Source: three-view drawing plus pictorial views. Frame: mm from the lowest corner of the part. A direction names the side the tool comes from. Give positions to 0.01 mm unless a question says otherwise; leave off trailing zeros. Loops run counter-clockwise (first coordinate to the right, second up) from the corner with the lowest first, then second, coordinate; pieces in that order, holes last. Notation, with made-up numbers: M -18,24 L -14,24 A32 ccw -14,58 Z; hole C 62,65 d8. An arc over 180 degrees is marked long. One line per item, written item: value. Start each with the question number.
(1) Section C-C on z = 16.5. Output: boundary loops of the cut face in (x, y), plus the area to 3 significant figures.
(2) Pin query (flat end, axial travel): P1, Ø4, axis at x = 6, y = 3, coming from the +Z side; P2, Ø2.5, axis at x = 5.5, y = 7, coming from the +Z side; P3, Ø2.5, axis at y = 1.5, z = 13, coming from the -X side; P4, Ø6, axis at x = 6.5, z = 11.5, coming from the -Y side. Return the tip coordinate at first contact, or that it passes through.
(3) Pull-direction query (Z, two-part tool) for the marked faces 1, 2, 3 and 4; classes: released by +Z, released by -Z, zero draft, split by the parting line, or undercut.
(4) Access query for the marked faces 5, 6, 7, 8 and 9. Directions: +Z, -Z, +X, -X, +Y, -Y. A direction counts if a zero-diameter tool reaches every point of the face in a straight line with its end or side. Return the directions, or none.
(5) Ray query, line 1 along Z through (x, y) = (3.5, 8) (1 decimal); line 2 along X through (y, z) = (4.5, 8.5); line 3 along Z through (x, y) = (10.5, 3.75). Return the intervals inside material, ascending. Write a range as from..to.
(6) Section B-B on x = 2. Output: boundary loops of the cut face in (y, z), plus the area to 3 significant figures.
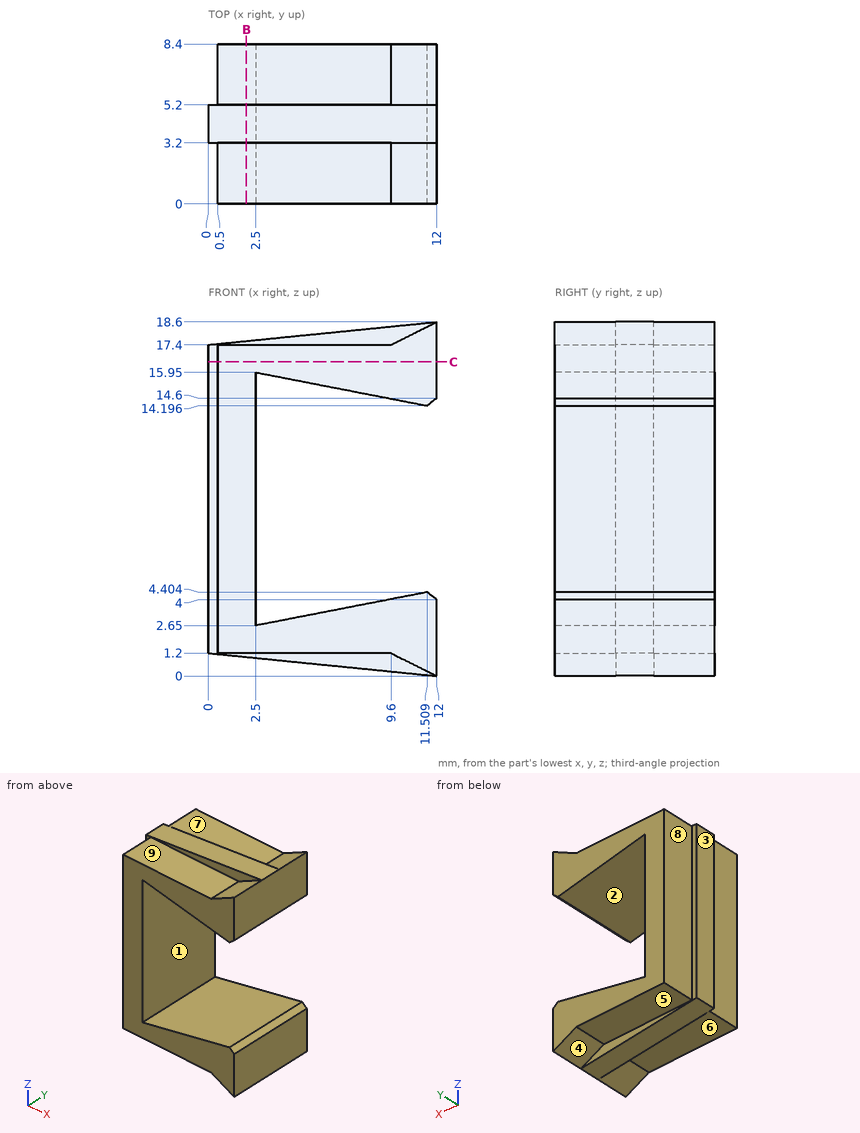
Output values:
1. outline: M 0,3.2 L 0.5,3.2 L 0.5,0 L 12,0 L 12,8.4 L 0.5,8.4 L 0.5,5.2 L 0,5.2 Z
1. area: 97.6 mm²
2. P1: stops at z = 18.2
2. P2: stops at z = 17.4
2. P3: stops at x = 0.5
2. P4: passes through
3. face 1: undercut
3. face 2: undercut
3. face 3: zero draft
3. face 4: released by -Z
4. face 5: -Z, -X, +Y
4. face 6: -Z, -X, -Y
4. face 7: +Z, -X, +Y
4. face 8: +Z, -Z, -X, +Y
4. face 9: +Z, -X, -Y
5. line 1: z = 1.2..2.8, 15.8..17.4
5. line 2: x = 0..2.5
5. line 3: z = 0.15..4.21, 14.39..18.45
6. outline: M 0,1.2 L 3.2,1.2 L 3.2,1 L 5.2,1 L 5.2,1.2 L 8.4,1.2 L 8.4,17.4 L 5.2,17.4 L 5.2,17.6 L 3.2,17.6 L 3.2,17.4 L 0,17.4 Z
6. area: 137 mm²
